Design review of the part built by this model. Coordinates are the model's own, in mm. A direction names the side the tool comes from. Round coordinates to 2 decimals unless told otherwise and drop trailing zeros. Loops run counter-clockwise (first coordinate to the right, second up) from the corner with the lowest first, then second, coordinate; pieces in that order, holes last. Notation, with made-up numbers: M -1,66 L 23,66 A20 cw 23,103 Z; hole C 34.5,31 d6. An arc over 180 degrees is marked long. Use a Markdown table: item, result.
from build123d import *

# Parameters (mm, degrees)
F0_R     = 26
F0_R_2   = 23.125
F3_R     = 26
F3_R_2   = 23.125
F3_R_3   = 22.5
F4_DEPTH = 1
F5_R     = 26
F5_R_2   = 23.125
F6_DEPTH = 25
F7_R     = 27.5
F7_R_2   = 26
F7_R_3   = 23.125
F8_DEPTH = 5
F7_R_4   = 30
F9_DEPTH = 35


with BuildPart() as f2:
    # F2: sweep along a path in F1
    with BuildLine(Plane.XZ) as f2_path:
        ThreePointArc((0, 0), (11.7157287525, -28.2842712475), (40, -40))
    # F0 (on Top) → F2 (sweep)
    with BuildSketch(Plane.XY):
        Circle(F0_R)
        Circle(F0_R_2, mode=Mode.SUBTRACT)
    sweep(path=f2_path.line)

    # F3 (on face) → F4 (join)
    with BuildSketch(Plane.XY):
        Circle(F3_R)
        Circle(F3_R_2, mode=Mode.SUBTRACT)
        Circle(F3_R_2)
        Circle(F3_R_3, mode=Mode.SUBTRACT)
    extrude(amount=F4_DEPTH)

    # F5 (on face) → F6 (join)
    with BuildSketch(Plane.XY.offset(1)):
        Circle(F5_R)
        Circle(F5_R_2, mode=Mode.SUBTRACT)
    extrude(amount=F6_DEPTH)

    # F7 (on face) → F8 (join)
    with BuildSketch(Plane.YZ.offset(40)):
        with Locations((0, -40)):
            Circle(F7_R)
        with Locations((0, -40)):
            Circle(F7_R_2, mode=Mode.SUBTRACT)
        with Locations((0, -40)):
            Circle(F7_R_2)
        with Locations((0, -40)):
            Circle(F7_R_3, mode=Mode.SUBTRACT)
    extrude(amount=F8_DEPTH)

    # F7 (on face) → F9 (join)
    with BuildSketch(Plane.YZ.offset(40)):
        with Locations((0, -40)):
            Circle(F7_R_4)
        with Locations((0, -40)):
            Circle(F7_R, mode=Mode.SUBTRACT)
    extrude(amount=F9_DEPTH)


solid = f2.part
1. Wall thickness on line 1 along Z through (x, y) = (56, 0); line 2 along Y through (x, z) = (0, 17) (3 decimals); line 3 along X through (y, z) = (10, -12): over which ranges is each line inside the solid? List them lowest first. Write a range as from..to.
Check values:
| item | result |
|---|---|
| line 1 | z = -70..-67.5, -12.5..-10 |
| line 2 | y = -26..-23.125, 23.125..26 |
| line 3 | x = -22.86..-19.66, 25.08..29.42, 40..75 |
2. Take a section at C-C on z = 16. Give the boundary of the cut face in (x, y) (3 decimals), and give its area (3 significant figures).
Check values:
| item | result |
|---|---|
| outline | C 0,0 d52; hole C 0,0 d46.25 |
| area | 444 mm² |
3. Insertion check: pin 1 (3 mm diameter, centred on y = 1.5, z = -30, fed in from -X); pin 2 (8 mm diameter, centred on x = -6, z = 2.5, fed in from -Y); pin 3 (1.5 mm diameter, centred on y = 11.5, z = 15, fed in from -X). Each pin has a flat end and moves straight along its axis. Give the tip position at first contact, or say it passes through.
Check values:
| item | result |
|---|---|
| pin 1 | stops at x = -19.49 |
| pin 2 | stops at y = -25.92 |
| pin 3 | stops at x = -23.67 |
4. Take a section at D-D on y = -8. Give the boundary of the cut face in (x, z).
Check values:
| item | result |
|---|---|
| outline | M -24.74,0 A64.74 ccw 40,-64.74 L 40,-68.91 L 75,-68.91 L 75,-66.31 L 45,-66.31 L 45,-61.7 L 40,-61.7 A61.7 cw -21.7,0 L -21.03,0 L -21.03,1 L -21.7,1 L -21.7,26 L -24.74,26 Z; M 21.03,0 L 21.7,0 A18.3 ccw 40,-18.3 L 45,-18.3 L 45,-13.69 L 75,-13.69 L 75,-11.09 L 40,-11.09 L 40,-15.26 A15.26 cw 24.74,0 L 24.74,26 L 21.7,26 L 21.7,1 L 21.03,1 Z |
5. Take a section at A-A on y = 0. Give the boundary of the cut face in (x, z) (3 decimals).
Check values:
| item | result |
|---|---|
| outline | M -26,0 A66 ccw 40,-66 L 40,-70 L 75,-70 L 75,-67.5 L 45,-67.5 L 45,-63.125 L 40,-63.125 A63.125 cw -23.125,0 L -22.5,0 L -22.5,1 L -23.125,1 L -23.125,26 L -26,26 Z; M 22.5,0 L 23.125,0 A16.875 ccw 40,-16.875 L 45,-16.875 L 45,-12.5 L 75,-12.5 L 75,-10 L 40,-10 L 40,-14 A14 cw 26,0 L 26,26 L 23.125,26 L 23.125,1 L 22.5,1 Z |
6. The part is to be moulded in two halves that separate along Z. For faces 1 (the face through (57.255, -6.503, -69.287)), 2 (the face through (45, -6, -17)), 3 (the face through (40, -9, -15)), say which applies: pulls with the +Z half, pulls with the -Z half, needs draft (parallel to the pull), parting line crosses it, or undercut.
Check values:
| item | result |
|---|---|
| face 1 | parting line crosses it |
| face 2 | undercut |
| face 3 | needs draft |
7. Machinability: for faces 4 (the face through (59.79, 12.69, -64.397)), 5 (the face through (75, 13.2, -64.3)), 6 (the face through (-23.23, -1.8, 26)), 7 (the face through (12.43, 19.5, 13.32)), 8 (the face through (5, -22.2, 0)), which of the approach directions +Z, -Z, +X, -X, +Y, -Y give a long, thin tool a straight path to every point of the face, cutting with its end or side? Answer none if there is none.
Check values:
| item | result |
|---|---|
| face 4 | +X |
| face 5 | +Z, -Z, +X, +Y, -Y |
| face 6 | +Z, +X, -X, +Y, -Y |
| face 7 | +Z |
| face 8 | none |
8. Take a section at B-B on x = 59.5. Give the boundary of the cut face in (y, z), and give its area (3 significant figures).
Check values:
| item | result |
|---|---|
| outline | C 0,-40 d60; hole C 0,-40 d55 |
| area | 452 mm² |
